Autodesk Inventor part; units mm, degrees
ref_plane "YZ Plane" through (0, 0, 0) normal (1, 0, 0) x (0, 1, 0)
ref_plane "XZ Plane" through (0, 0, 0) normal (0, 1, 0) x (-1, 0, 0)
ref_plane "XY Plane" through (0, 0, 0) normal (0, 0, 1) x (1, 0, 0)
ref_plane "Work Plane1" through (0, 0, 0) normal (0, 0, 1) x (1, 0, 0)
sketch "Sketch1" plane through (0, 0, 0) normal (0, 0, 1) x (1, 0, 0)
  circle A0 centre (25, -10) radius 1.45
  circle A1 centre (-25, -10) radius 1.45
  circle A2 centre (-25, 10) radius 1.45
  circle A3 centre (25, 10) radius 1.45
  circle A4 centre (-10, -25) radius 1.45
  circle A5 centre (-10, 25) radius 1.45
  circle A6 centre (10, 25) radius 1.45
  circle A7 centre (10, -25) radius 1.45
  circle A8 centre (-25, 25) radius 2.325
  circle A9 centre (25, -25) radius 2.325
  circle A10 centre (-25, -25) radius 2.325
  circle A11 centre (25, 25) radius 2.325
  line L0 (28, 30) -> (30, 28)
  line L1 (28, 30) -> (-28, 30)
  line L2 (-30, 28) -> (-28, 30)
  line L3 (-30, 28) -> (-30, -28)
  line L4 (-28, -30) -> (-30, -28)
  line L5 (-28, -30) -> (28, -30)
  line L6 (30, -28) -> (28, -30)
  line L7 (30, -28) -> (30, 28)
  circle A12 centre (-17.5, -17.5) radius 1.95
  circle A13 centre (17.5, 17.5) radius 1.95
  circle A14 centre (17.5, -17.5) radius 1.95
  circle A15 centre (-17.5, 17.5) radius 1.95
  circle A16 centre (0, 0) radius 7.5
  line L8 (30, -30) -> (-5, -30)
  line L9 (-5, -30) -> (-5, 5)
  line L10 (-5, 5) -> (30, 5)
  line L11 (30, 5) -> (30, -30)
  point P0 (0, 0)
  dimension "d0" = 35
  dimension "d1" = 35
extrude "Extrusion1" add sketch "Sketch1" along normal blind 7 contours A0 | A7 | A9 | L7 L6 L5 L9 A16 L10 | A16 L9 L10 | A14 picked at (1.7753, -1.9143)
sketch "Sketch2" plane through (0, 0, 7) normal (0, 0, 1) x (1, 0, 0)
  line L0 (9.7965, -11.8691) -> (15.0465, -11.8691)
  line L1 (-5, 5) -> (-5, -30)
  line L2 (-5, -30) -> (28, -30)
  line L3 (28, -30) -> (30, -28)
  line L4 (30, -28) -> (30, 5)
  line L5 (30, 5) -> (-5, 5)
  circle A0 centre (12.5, -12.5) radius 17.5
  line L6 (25, -25) -> (0, -25)
  line L7 (0, -25) -> (0, 0)
  line L8 (0, 0) -> (25, 0)
  line L9 (25, 0) -> (25, -25)
  line L10 (25, -25) -> (0, 0) construction
  line L11 (0, -25) -> (25, 0) construction
  dimension "d4" = 25
  dimension "d5" = 25
hole "Hole1" at (25, 0, 7) at (0, -25, 7) at (0, 0, 7) at (25, -25, 7) direction (0, 0, -1) diameter 3 end through all counterbore diameter 6 counterbore depth 3
sketch "Sketch3" plane through (0, 0, 7) normal (0, 0, 1) x (1, 0, 0)
  circle A0 centre (18.5383, 7.9631) radius 1.4 construction
  circle A1 centre (8.5565, 1.2345) radius 2.95 construction
  circle A2 centre (8.5565, -23.0142) radius 2.95 construction
  circle A3 centre (29.5565, -10.8899) radius 2.95 construction
  line L0 (4.5565, -28.3465) -> (33.5565, -28.3465) construction
  line L1 (4.5565, 11.2345) -> (4.5565, -28.3465) construction
  line L2 (33.5565, 11.2345) -> (4.5565, 11.2345) construction
  line L3 (33.5565, -28.3465) -> (33.5565, 11.2345) construction
  line L4 (-5, 5) -> (-5, -30) construction
  line L5 (30, 5) -> (-5, 5) construction
  line L6 (30, -28) -> (30, 5) construction
  circle A4 centre (12.5, -12.5) radius 17.5 construction
  line L7 (26.5, -12.5) -> (5.5, -24.6244) construction
  line L8 (5.5, -24.6244) -> (5.5, -0.3756) construction
  line L9 (5.5, -0.3756) -> (26.5, -12.5) construction
  point P0 (0, 0)
  dimension "d13" = 12.1244
  dimension "d14" = 21
  dimension "d15" = 21
hole "Hole2" at (26.5, -12.5, 7) at (5.5, -24.6244, 7) at (5.5, -0.3756, 7) direction (0, 0, -1) diameter 2.8 end through all
properties part number "30_cellSTORM_UC2_Chip_holder_base"
CAD build for the part. Positions are in the model's coordinates, mm. A direction names the side the tool comes from. Coordinates: 2 decimals unless noted, no trailing zeros. Order: outer loops, then holes, each group sorted by start corner. A loop starts at its lowest first (then second) coordinate and runs counter-clockwise, first axis right, second up. Notation, with made-up numbers: M -34,88 L 7,88 A22 ccw 7,115 Z; hole C 77,77 d6. An arc over 180 degrees is marked long. Write each question's results on one line, items separated by ' | '. Start each with the question number.
Q1. Cut at C-C (y = 0). List the corners of the cut face in (x, z).
Q2. Flat gauge pins, fed straight in: P1, Ø1.7, axis at x = 5.5, y = -0.38, coming from the +Z side; P2, Ø5.5, axis at x = 25, y = -25, coming from the +Z side. Where does each tip first touch, or does it go through?
Q3. Cut at D-D (x = 0). List the corners of the cut face in (y, z).
Q4. Pull direction X, two halves, no side cores. Call faces 1 (the cylindrical face through (27.35, -11.39, 3.45)), 2 (the flat face through (30, -12, 3)), 3 (the flat face through (12, -12, 7)), 4 (the flat face through (-5, -13, 3)): +X half, -X half, draft (parallel to the pull), parting line (faces both ways), or undercut.
Q5. Drill centre lines: probe 1 along Y at (x, z) = (0, 6.4); probe 2 along Y at (x, z) = (0, 1.1); probe 3 along X at (y, z) = (-24.5, 4.75). Where is each one in solid material? Low to high. Write a range as from..to.
Q6. Cut at B-B (x = 5.5). List the corners of the cut face in (y, z).
Q7. Cut at A-A (z = 2). List the corners of the cut face in (x, y).
Q8. Which spindle directions (+Z, -Z, +X, -X, +Y, -Y) get a long thin tool onto all of the face, cutting with end or side? Do faces 5 (the flat face through (26.3, -26.3, 4)), 6 (the cylindrical face through (5.438, -23.226, 3.451)). Say none if no direction does.
Found:
1) outline: M -5,0 L -1.5,0 L -1.5,4 L -3,4 L -3,7 L -5,7 Z; M 1.5,0 L 4.15,0 L 4.15,7 L 3,7 L 3,4 L 1.5,4 Z; M 6.85,0 L 23.5,0 L 23.5,4 L 22,4 L 22,7 L 6.85,7 Z; M 26.5,0 L 30,0 L 30,7 L 28,7 L 28,4 L 26.5,4 Z
2) P1: through | P2: z = 4
3) outline: M -30,0 L -26.5,0 L -26.5,4 L -28,4 L -28,7 L -30,7 Z; M -23.5,0 L -1.5,0 L -1.5,4 L -3,4 L -3,7 L -22,7 L -22,4 L -23.5,4 Z; M 1.5,0 L 5,0 L 5,7 L 3,7 L 3,4 L 1.5,4 Z
4) face 1: undercut | face 2: +X half | face 3: draft | face 4: -X half
5) probe 1: -30..-28, -22..-3, 3..5 | probe 2: -30..-26.5, -23.5..-1.5, 1.5..5 | probe 3: -5..-2.96, 2.96..4.11, 6.89..22.04, 27.96..30
6) outline: M -30,0 L -26.02,0 L -26.02,7 L -30,7 Z; M -23.22,0 L -1.78,0 L -1.78,7 L -23.22,7 Z; M 1.02,0 L 5,0 L 5,7 L 1.02,7 Z
7) outline: M -5,-30 L 28,-30 L 30,-28 L 30,5 L -5,5 Z; hole C 0,-25 d3; hole C 0,0 d3; hole C 5.5,-24.62 d2.8; hole C 5.5,-0.38 d2.8; hole C 25,-25 d3; hole C 25,0 d3; hole C 26.5,-12.5 d2.8
8) face 5: +Z | face 6: +Z, -Z
